Build history of the part. All positions in model axes, mm. Face numbers are marked on the shaded views. A direction names the side the tool comes from. Give positions to 0.01 mm unless a question says otherwise; leave off trailing zeros. Loops run counter-clockwise (first coordinate to the right, second up) from the corner with the lowest first, then second, coordinate; pieces in that order, holes last. Notation, with made-up numbers: (51, 59) -> (63, 59) arc R21 cw to (63, 78) -> close; hole circle Ø10 at (44.5, -18). An arc over 180 degrees is marked (long way). Answer as a JSON object with one key per item and string values. Group by question number.
Q1. Band-saw the part on A-A, the plane x = 0. Count the separate pieces of the cut face and the enclosed holes in it, plus the area to 3 significant figures.
Q2. Wall check: probe 1 along Z at (x, y) = (0, 1.25) (3 decimals); probe 2 along Z at (x, y) = (0, -6.5); probe 3 along X at (y, z) = (-4.5, -0.25). Give the ranges that are in metal, low to high. Write a range as from..to.
Q3. Band-saw the part on B-B, the plane z = 3. Write the cut outline in (x, y).
Q4. Drop flat-ended pins along their axis: pin 1 (4 mm diameter, centred on x = -3, z = 1, fed in from -Y); pin 2 (3 mm diameter, centred on x = 0.5, y = 3, fed in from +Z); pin 3 (3 mm diameter, centred on x = 3.5, y = -3.5, fed in from -Z); pin 4 (5 mm diameter, centred on x = 0, z = 0, fed in from -Y). Give the stop position or say it passes through.
Q5. Band-saw the part on D-D, the plane x = -3.5. Write the cut outline in (y, z) (3 decimals), plus the area to 3 significant figures.
Q6. Two-plate mould, pull along X, no slides. Class the marked faces 1, 2, 3 and 4: pulls with the +X half, pulls with the -X half, needs draft (parallel to the pull), parting line crosses it, or undercut.
Q7. Tool access for the marked faces 5, 6 and 7: list every direction of +Z, -Z, +X, -X, +Y, -Y with a clear straight run to the whole face (end or side of a thin tool).
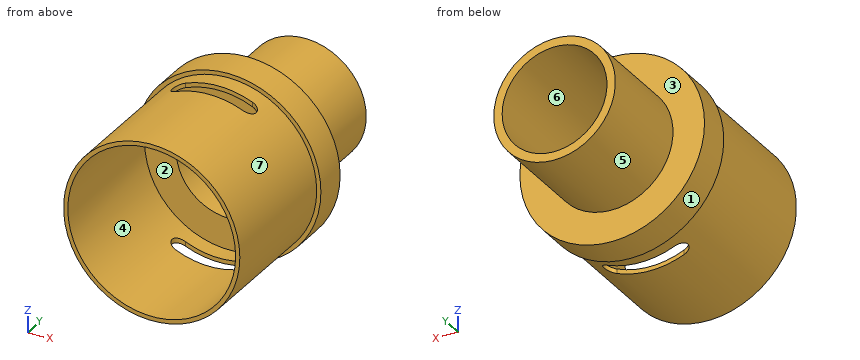
from build123d import *

# Parameters (mm, degrees)
F0_R     = 4.6
F0_R_2   = 3.965
F1_DEPTH = 7.62
F0_R_3   = 6.985
F0_R_4   = 6.35
F2_DEPTH = 2.54
F3_DEPTH = 12.7
F5_R     = 6.985
F5_R_2   = 6.6675
F6_DEPTH = 10.16
F7_DEPTH = 6.82625


# Not quite as in the source:
# - a feature names something its author has since deleted; it is built from what else it names


with BuildPart() as f1:
    # F0 (on Front) → F1 (new body)
    with BuildSketch(Plane.XZ):
        Circle(F0_R)
        Circle(F0_R_2, mode=Mode.SUBTRACT)
    extrude(amount=-F1_DEPTH)

    # F0 (on Front) → F2 (join)
    with BuildSketch(Plane.XZ):
        Circle(F0_R_3)
        Circle(F0_R_4, mode=Mode.SUBTRACT)
        Circle(F0_R_4)
        Circle(F0_R, mode=Mode.SUBTRACT)
        Circle(F0_R)
        Circle(F0_R_2, mode=Mode.SUBTRACT)
    extrude(amount=F2_DEPTH)

    # F0 (on Front) → F3 (join)
    with BuildSketch(Plane.XZ):
        Circle(F0_R_3)
        Circle(F0_R_4, mode=Mode.SUBTRACT)
    extrude(amount=F3_DEPTH)

    # F5 (on face) → F6 (cut)
    with BuildSketch(Plane.XZ.offset(12.7)):
        Circle(F5_R)
        Circle(F5_R_2, mode=Mode.SUBTRACT)
    extrude(amount=-F6_DEPTH, mode=Mode.SUBTRACT)

    # F4 (on Top) → F7 (cut, symmetric)
    with BuildSketch(Plane.XY):
        with BuildLine():
            Line((2.54, -3.81), (0, -3.81))
            Line((0, -3.81), (-2.54, -3.81))
            ThreePointArc((-2.54, -3.81), (-3.175, -4.445), (-2.54, -5.08))
            Line((-2.54, -5.08), (0, -5.08))
            Line((0, -5.08), (2.54, -5.08))
            ThreePointArc((2.54, -5.08), (3.175, -4.445), (2.54, -3.81))
        make_face()
    extrude(amount=F7_DEPTH, both=True, mode=Mode.SUBTRACT)


solid = f1.part
Worked answers:
{
 "1": {"separate pieces": "4", "enclosed holes": "0", "area": "30.7 mm2"},
 "2": {"probe 1": "-4.6..-3.965, 3.965..4.6", "probe 2": "-6.67..-6.35, 6.35..6.67", "probe 3": "-6.66..-6.35, 6.35..6.66"},
 "3": {"outline": "(-6.31, -2.54) -> (-5.95, -2.54) -> (-5.95, -12.7) -> (-5.6, -12.7) -> (-5.6, -2.54) -> (-2.59, -2.54) -> (-2.59, 7.62) -> (-3.49, 7.62) -> (-3.49, 0) -> (-6.31, 0) -> close; (2.59, -2.54) -> (5.6, -2.54) -> (5.6, -12.7) -> (5.95, -12.7) -> (5.95, -2.54) -> (6.31, -2.54) -> (6.31, 0) -> (3.49, 0) -> (3.49, 7.62) -> (2.59, 7.62) -> close"},
 "4": {"pin 1": "y = -2.54", "pin 2": "z = 4.6", "pin 3": "z = -6.58", "pin 4": "through"},
 "5": {"outline": "(-12.7, -5.675) -> (-2.54, -5.675) -> (-2.54, -6.045) -> (0, -6.045) -> (0, -2.985) -> (7.62, -2.985) -> (7.62, -1.863) -> (-2.54, -1.863) -> (-2.54, -5.298) -> (-12.7, -5.298) -> close; (-12.7, 5.298) -> (-2.54, 5.298) -> (-2.54, 1.863) -> (7.62, 1.863) -> (7.62, 2.985) -> (0, 2.985) -> (0, 6.045) -> (-2.54, 6.045) -> (-2.54, 5.675) -> (-12.7, 5.675) -> close", "area": "46.0 mm2"},
 "6": {"face 1": "parting line crosses it", "face 2": "undercut", "face 3": "needs draft", "face 4": "undercut"},
 "7": {"face 5": "+Y", "face 6": "+Y, -Y", "face 7": "-Y"}
}
